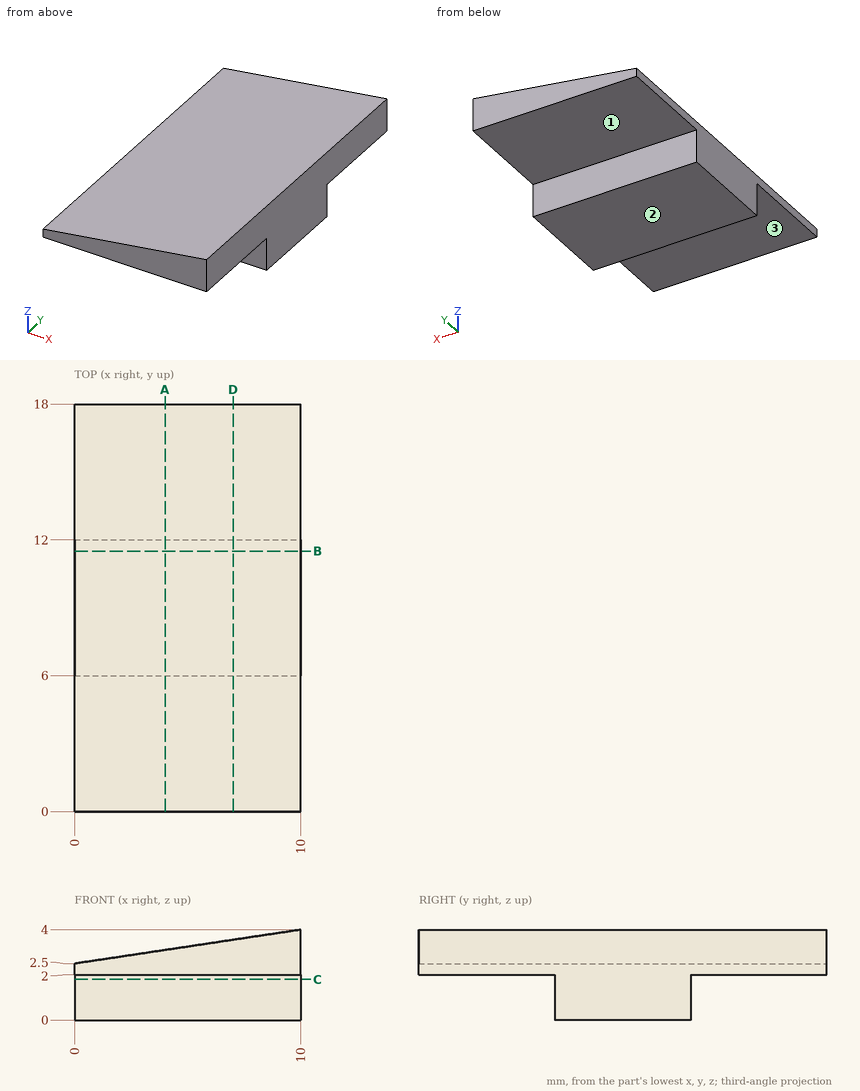
Study the drawing (mm; zero at the part's minimum x, y, z) and answer. A direction names the side the tool comes from. Round coordinates to 2 decimals unless told otherwise and drop trailing zeros. Order: outer loops, then holes, each group sorted by start corner. A loop starts at its lowest first (then second) coordinate and runs counter-clockwise, first axis right, second up. Notation, with made-up numbers: M 55,86.5 L 111,86.5 A22 ccw 111,125.5 Z; hole C -20,25.25 d6. An arc over 180 degrees is marked long. One line per item, written item: value.
Q1. Find section A-A on x = 4. Write down the section's boundary in (y, z), then the cut area to 3 significant figures.
Derived:
outline: M 0,2 L 6,2 L 6,0 L 12,0 L 12,2 L 18,2 L 18,3.1 L 0,3.1 Z
area: 31.8 mm²
Q2. Find section C-C on z = 1.8. Write down the section's boundary in (x, y).
Derived:
outline: M 0,6 L 10,6 L 10,12 L 0,12 Z
Q3. Flat-ended cylindrical pins translate along their axes: pin 1 (3 mm diameter, centred on x = 4, y = 1.5, fed in from -Z); pin 2 (1 mm diameter, centred on x = 4, z = 1, fed in from +Y). Find the tip coordinate at first contact, or state that the pin passes through.
Derived:
pin 1: z = 2
pin 2: y = 12
Q4. Find section B-B on y = 11.5. Write down the section's boundary in (x, z), then the cut area to 3 significant figures.
Derived:
outline: M 0,0 L 10,0 L 10,4 L 0,2.5 Z
area: 32.5 mm²
Q5. Find section D-D on x = 7. Write down the section's boundary in (y, z).
Derived:
outline: M 0,2 L 6,2 L 6,0 L 12,0 L 12,2 L 18,2 L 18,3.55 L 0,3.55 Z
Q6. Straight lines are drawn through the part: line 1 (Y direction, x = 8, z = 0.9); line 2 (Z direction, x = 9.25, y = 7.5); line 3 (Z direction, x = 1.25, y = 8). For each, find the intervals that lie inside material, in ascending order.
Derived:
line 1: 6 to 12
line 2: 0 to 3.89
line 3: 0 to 2.69
Q7. For the marked faces 1, 2 and 3, determine the directions among +Z, -Z, +X, -X, +Y, -Y from which every point of the face is accessible in a straight line to the end or side of a thin tool.
Derived:
face 1: -Z, +X, -X, +Y
face 2: -Z, +X, -X, +Y, -Y
face 3: -Z, +X, -X, -Y
